from build123d import *

# Parameters (mm, degrees)
F0_R     = 70
F0_R_2   = 3
F0_R_3   = 1.15
F1_DEPTH = 3


with BuildPart() as f1:
    # F0 (on Top) → F1 (new body)
    with BuildSketch(Plane.XY):
        Circle(F0_R)
        with Locations((-35.355339, -35.355339)):
            Circle(F0_R_2, mode=Mode.SUBTRACT)
        with Locations((-19.134172, -46.193977)):
            Circle(F0_R_2, mode=Mode.SUBTRACT)
        with Locations((-46.193977, -19.134172)):
            Circle(F0_R_2, mode=Mode.SUBTRACT)
        with Locations((0, -50)):
            Circle(F0_R_2, mode=Mode.SUBTRACT)
        with Locations((19.134172, -46.193977)):
            Circle(F0_R_2, mode=Mode.SUBTRACT)
        with Locations((35.355339, -35.355339)):
            Circle(F0_R_2, mode=Mode.SUBTRACT)
        with BuildLine():
            ThreePointArc((30.103986, -30), (0, -42.5), (-30.103986, -30))
            Line((-30.103986, -30), (-42.083251, -30))
            ThreePointArc((-42.083251, -30), (-45.083251, -27), (-42.083251, -24))
            Line((-42.083251, -24), (-35.07492, -24))
            Line((-35.07492, -24), (35.07492, -24))
            Line((35.07492, -24), (42.083251, -24))
            ThreePointArc((42.083251, -24), (45.083251, -27), (42.083251, -30))
            Line((42.083251, -30), (30.103986, -30))
        make_face(mode=Mode.SUBTRACT)
        with Locations((0, -8)):
            Circle(F0_R_3, mode=Mode.SUBTRACT)
        with Locations((46.193977, -19.134172)):
            Circle(F0_R_2, mode=Mode.SUBTRACT)
        with Locations((-50, 0)):
            Circle(F0_R_2, mode=Mode.SUBTRACT)
        with Locations((-46.193977, 19.134172)):
            Circle(F0_R_2, mode=Mode.SUBTRACT)
        with Locations((-8, 0)):
            Circle(F0_R_3, mode=Mode.SUBTRACT)
        with Locations((-35.355339, 35.355339)):
            Circle(F0_R_2, mode=Mode.SUBTRACT)
        with Locations((-19.134172, 46.193977)):
            Circle(F0_R_2, mode=Mode.SUBTRACT)
        with Locations((8, 0)):
            Circle(F0_R_3, mode=Mode.SUBTRACT)
        with Locations((0, 8)):
            Circle(F0_R_3, mode=Mode.SUBTRACT)
        with Locations((50, 0)):
            Circle(F0_R_2, mode=Mode.SUBTRACT)
        with Locations((46.193977, 19.134172)):
            Circle(F0_R_2, mode=Mode.SUBTRACT)
        with Locations((0, 50)):
            Circle(F0_R_2, mode=Mode.SUBTRACT)
        with Locations((19.134172, 46.193977)):
            Circle(F0_R_2, mode=Mode.SUBTRACT)
        with Locations((35.355339, 35.355339)):
            Circle(F0_R_2, mode=Mode.SUBTRACT)
    extrude(amount=F1_DEPTH)


solid = f1.part
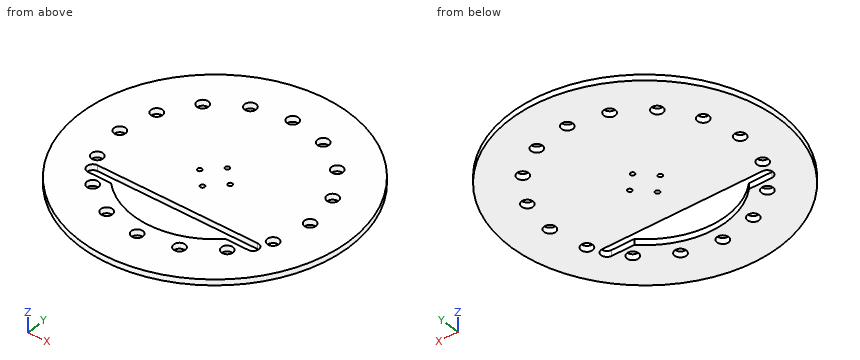
Can you work these out from the model? Positions are in its coordinate system, mm. Coordinates: 2 decimals unless noted, no trailing zeros. Order: outer loops, then holes, each group sorted by start corner. A loop starts at its lowest first (then second) coordinate and runs counter-clockwise, first axis right, second up. Notation, with made-up numbers: M 35.5,-35 L 87.5,-35 A24 ccw 87.5,-23 Z; hole C -14,78 d10. An arc over 180 degrees is marked long. Write item = value, one per line.
(1) I need wall thicknesses on line 1 along Y through (x, z) = (0, 2.15); line 2 along Y through (x, z) = (-2, 1); line 3 along X through (y, z) = (-44, 2.5). Which ranges of each line are inside material? Lowest first, please. Write a range as [from, to].
Results are:
line_1 = [-70, -53], [-47, -42.5], [-24, -9.15], [-6.85, 6.85], [9.15, 47], [53, 70]
line_2 = [-69.97, -52.24], [-47.76, -42.45], [-24, 47.76], [52.24, 69.97]
line_3 = [-54.44, -21.18], [-17.09, 17.09], [21.18, 54.44]
(2) Suppose I cut it at B-B on x = 55. Please give me the cut outline in (y, z), plus the area to 3 significant figures.
Results are:
outline = M -43.3,0 L 43.3,0 L 43.3,3 L -43.3,3 Z
area = 260 mm2
(3) For pin 1 Ø3.5 at (x, y) = (35.36, -35.36) entering from -Z; pin 2 Ø1 at (x, z) = (-11, 2.5) entering from -Y, each with a flat end and sliding along its axis, tell me the tip position at first contact or that it passes through.
Results are:
pin_1 = through
pin_2 = -69.21
(4) Suppose I cut it at A-A on z = 2.15. State how many separate pieces and enclosed holes the cut face has, plus the area to 3 significant figures.
Results are:
separate_pieces = 1
enclosed_holes = 21
area = 13,900 mm2
(5) Suppose I cut it at C-C on y = -61. Please give me the cut outline in (x, z).
Results are:
outline = M -34.34,0 L 34.34,0 L 34.34,3 L -34.34,3 Z
